```python
from build123d import *

# Parameters (mm, degrees)
SKETCH_1_W               = 20
SKETCH_1_H               = 23
EXTRUDE_1_DEPTH          = 34
CUT_EXTRUDE_1_DEPTH      = 10
CUT_EXTRUDE_1_DEPTH_BACK = 34
SKETCH_2_R               = 0.8
SKETCH_3_R               = 8
EXTRUDE_2_DEPTH          = 3
SKETCH_4_R               = 0.75
CUT_EXTRUDE_2_DEPTH      = 3


with BuildPart() as part:
    # 草图1 → 凸台-拉伸1 (new body)
    with BuildSketch(Plane(origin=(0, 0, 0), x_dir=(0, 0, -1), z_dir=(1, 0, 0))):
        Rectangle(SKETCH_1_W, SKETCH_1_H)
    extrude(amount=EXTRUDE_1_DEPTH)

    # 草图2 → 切除-拉伸1 (cut, two sides: drawn at the far end of the back side and taken through both)
    with BuildSketch(Plane(origin=(0, -11.5, 0), x_dir=(-1, 0, 0), z_dir=(0, -1, 0)).offset(-CUT_EXTRUDE_1_DEPTH_BACK)):
        with Locations(Location((-2, -8, 0), (0, 0, 270))):
            Circle(SKETCH_2_R)
        with Locations(Location((-2, 8, 0), (0, 0, 270))):
            Circle(SKETCH_2_R)
    extrude(amount=CUT_EXTRUDE_1_DEPTH + CUT_EXTRUDE_1_DEPTH_BACK, mode=Mode.SUBTRACT)

    # 草图3 → 凸台-拉伸2 (add)
    with BuildSketch(Plane(origin=(0, 11.5, 0), x_dir=(1, 0, 0), z_dir=(0, 1, 0))):
        with Locations(Location((25, 0, 0), (0, 0, 90))):
            Circle(SKETCH_3_R)
    extrude_2 = extrude(amount=EXTRUDE_2_DEPTH)

    # 镜向1: 凸台-拉伸2 across plane
    add(extrude_2.mirror(Plane.ZX))

    # 草图4 → 切除-拉伸2 (cut)
    with BuildSketch(Plane(origin=(0, 14.5, 0), x_dir=(1, 0, 0), z_dir=(0, 1, 0))):
        with Locations(Location((25, -6, 0), (0, 0, 270))):
            Circle(SKETCH_4_R)
        with Locations((45.5, 14.5)):
            Circle(SKETCH_4_R)
        with Locations((25, 35)):
            Circle(SKETCH_4_R)
        with Locations((4.5, 14.5)):
            Circle(SKETCH_4_R)
        with Locations(Location((19, 0, 0), (0, 0, 270))):
            Circle(SKETCH_4_R)
        with Locations(Location((25, 6, 0), (0, 0, 270))):
            Circle(SKETCH_4_R)
        with Locations(Location((31, 0, 0), (0, 0, 270))):
            Circle(SKETCH_4_R)
    cut_extrude_2 = extrude(amount=-CUT_EXTRUDE_2_DEPTH, mode=Mode.SUBTRACT)

    # 镜向2: 切除-拉伸2 across plane
    add(cut_extrude_2.mirror(Plane.ZX), mode=Mode.SUBTRACT)


solid = part.part
```
Geometry check sheet. Reference: the model listing, model coordinates, mm. A direction names the side the tool comes from. Coordinates: 2 decimals unless noted, no trailing zeros. Write each loop counter-clockwise with the first axis right and the second up, starting at its lowest first coordinate (ties: lowest second). Pieces come first, ordered by that corner, then holes. Notation, with made-up numbers: M 4.25,24 L 23.25,24 A14 cw 23.25,44 Z; hole C 19.25,69.25 d6. An arc over 180 degrees is marked long. One line per item, written item: value. Start each with the question number.
(1) Release check for a two-part mould opening along Z. For faces 1 (the face through (29.868, 12.979, 6.349)), 2 (the face through (24.268, 13.021, 5.837)), 3 (the face through (13, -11.5, 0)) record: released by +Z, released by -Z, zero draft, split by the parting line, or undercut.
(2) Tool access check on faces 4 (the face through (19, 11.5, 0)), 5 (the face through (31, -11.5, 0)), 6 (the face through (17, 0, 10)). Record the directions out of +Z, -Z, +X, -X, +Y, -Y that give a thin tool (end or side, any length) a straight path to the whole face; none if there is none.
(3) Sectioned sample at B-B, the plane z = 0. Enter the section's corners in (x, y).
(4) Scan lines: line 1 along X through (y, z) = (-13.45, 0); line 2 along X through (y, z) = (5.75, -8); line 3 along Y through (x, z) = (16, 1.75). Record each from-to range of solid material in increasing order. Write a range as [from, to].
(5) Sectioned sample at D-D, the plane x = 19. Enter the section's corners in (y, z), and give its area (3 significant figures).
(6) Sectioned sample at C-C, the plane x = 25. Enter the section's corners in (y, z), and give its area (3 significant figures).
(7) Depth check by flat-ended pin: pin 1 (2.5 mm diameter, centred on x = 2, z = -8, fed in from -Y); pin 2 (6 mm diameter, centred on x = 7, z = 2, fed in from +Y). Enter the tip coordinate at first touch or a pass-through.
(8) Sectioned sample at A-A, the plane x = 2. Enter the section's corners in (y, z).
Filled sheet:
1. face 1: split by the parting line
1. face 2: undercut
1. face 3: zero draft
2. face 4: +Y
2. face 5: -Y
2. face 6: +Z, +X, -X, +Y, -Y
3. outline: M 0,-11.5 L 17,-11.5 L 17,-14.5 L 18.25,-14.5 L 18.25,-11.5 L 19.75,-11.5 L 19.75,-14.5 L 30.25,-14.5 L 30.25,-11.5 L 31.75,-11.5 L 31.75,-14.5 L 33,-14.5 L 33,-11.5 L 34,-11.5 L 34,11.5 L 33,11.5 L 33,14.5 L 31.75,14.5 L 31.75,11.5 L 30.25,11.5 L 30.25,14.5 L 19.75,14.5 L 19.75,11.5 L 18.25,11.5 L 18.25,14.5 L 17,14.5 L 17,11.5 L 0,11.5 Z
4. line 1: [17, 18.25], [19.75, 30.25], [31.75, 33]
4. line 2: [0, 1.2], [2.8, 34]
4. line 3: [-11.5, 11.5]
5. outline: M -14.5,-5.29 L -11.5,-5.29 L -11.5,-10 L 11.5,-10 L 11.5,-5.29 L 14.5,-5.29 L 14.5,-0.75 L 11.5,-0.75 L 11.5,0.75 L 14.5,0.75 L 14.5,5.29 L 11.5,5.29 L 11.5,10 L -11.5,10 L -11.5,5.29 L -14.5,5.29 L -14.5,0.75 L -11.5,0.75 L -11.5,-0.75 L -14.5,-0.75 Z
5. area: 514 mm²
6. outline: M -14.5,-8 L -11.5,-8 L -11.5,-10 L 11.5,-10 L 11.5,-8 L 14.5,-8 L 14.5,-6.75 L 11.5,-6.75 L 11.5,-5.25 L 14.5,-5.25 L 14.5,5.25 L 11.5,5.25 L 11.5,6.75 L 14.5,6.75 L 14.5,8 L 11.5,8 L 11.5,10 L -11.5,10 L -11.5,8 L -14.5,8 L -14.5,6.75 L -11.5,6.75 L -11.5,5.25 L -14.5,5.25 L -14.5,-5.25 L -11.5,-5.25 L -11.5,-6.75 L -14.5,-6.75 Z
6. area: 538 mm²
7. pin 1: y = -11.5
7. pin 2: y = 11.5
8. outline: M -11.5,-10 L 11.5,-10 L 11.5,-8.8 L -11.5,-8.8 Z; M -11.5,-7.2 L 11.5,-7.2 L 11.5,7.2 L -11.5,7.2 Z; M -11.5,8.8 L 11.5,8.8 L 11.5,10 L -11.5,10 Z
